The figure shows three views and two pictorial views of one solid part (mm, origin at its lowest corner). Answer the questions. A direction names the side the tool comes from. Coordinates: 2 decimals unless noted, no trailing zeros. Write each loop counter-clockwise with the first axis right and the second up, starting at its lowest first coordinate (ties: lowest second). Pieces come first, ordered by that corner, then holes.
Item 1: A tool of negligible diameter and unlimited length cuts with its end or side. For the marked faces 1 and 2, from which of +Z, -Z, +X, -X, +Y, -Y can it reach the whole face along a straight path? Write none if from no direction.
Item 2: Section C-C (z = 3.5) is taken. Give the vertices of the cut face in (x, y), then the cut area to 3 significant figures.
Item 3: Straight lines are drawn through the part: probe 1 along Y at (x, z) = (3.5, 1.1); probe 2 along X at (y, z) = (12.25, 3) (1 decimal); probe 3 along Z at (x, y) = (3.8, 15.25). For each, find the intervals that lie inside material, in ascending order.
Item 4: Section A-A (y = 9) is taken. Give the vertices of the cut face in (x, z), then the cut area to 3 significant figures.
Item 5: Section D-D (z = 0.4) is taken. Give the vertices of the cut face in (x, y).
Item 6: Section B-B (x = 3) is taken. Give the vertices of the cut face in (y, z).
Item 7: Each of these flat-tipped pins is pushed along its axis until it touches: P1, Ø2.5, axis at x = 3, z = 2.6, coming from the -Y side; P2, Ø1.5, axis at x = 2.5, z = 3, coming from the +Y side. Where does it stop, or does it pass through?
Item 8: Determine the mould class of the marked faces 3, 4 and 5 for opening direction Z: released by +Z, released by -Z, zero draft, split by the parting line, or undercut.
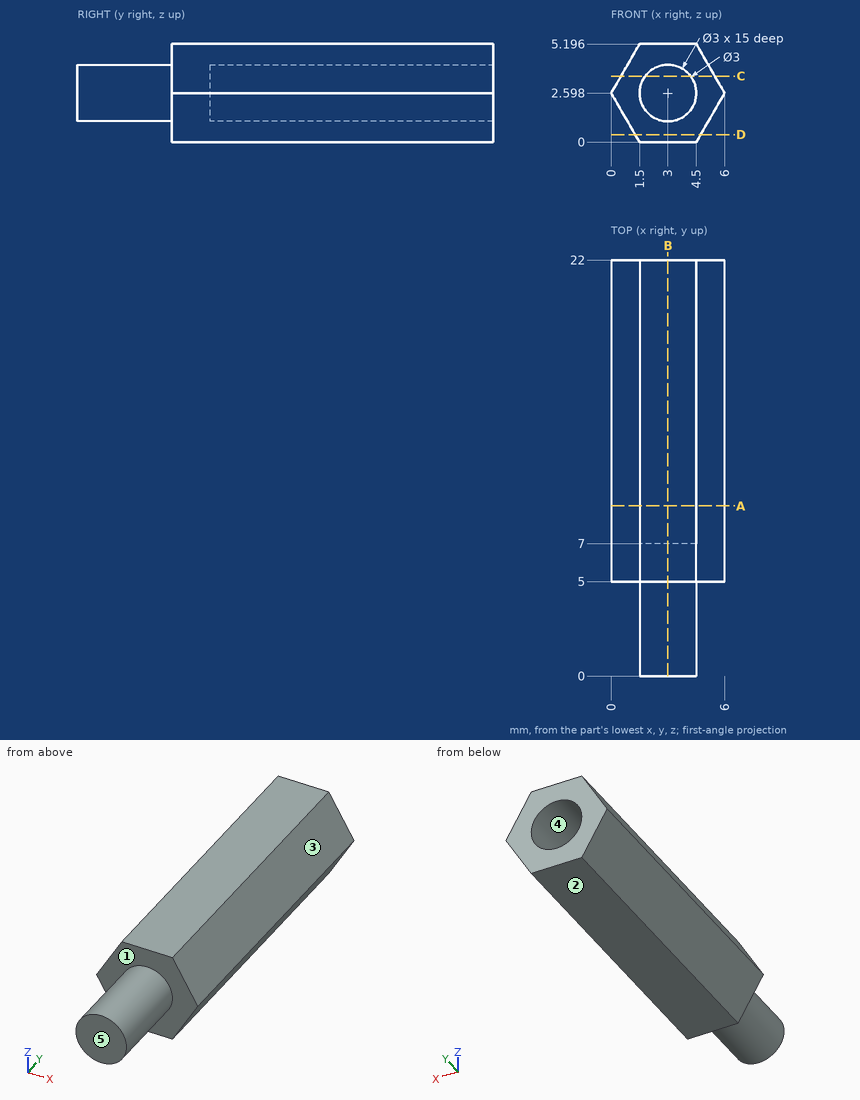
Established:
1. face 1: -Y
1. face 2: -Z, +X, -X, +Y, -Y
2. outline: (0.52, 5) - (1.8, 5) - (1.8, 0) - (4.2, 0) - (4.2, 5) - (5.48, 5) - (5.48, 22) - (4.2, 22) - (4.2, 7) - (1.8, 7) - (1.8, 22) - (0.52, 22) - close
2. area: 60.3 mm2
3. probe 1: y = 5 to 22
3. probe 2: x = 0.2 to 1.6, 4.4 to 5.8
3. probe 3: z = 0 to 1.33, 3.87 to 5.2
4. outline: (0, 2.6) - (1.5, 0) - (4.5, 0) - (6, 2.6) - (4.5, 5.2) - (1.5, 5.2) - close; hole circle Ø3 at (3, 2.6)
4. area: 16.3 mm2
5. outline: (1.27, 5) - (4.73, 5) - (4.73, 22) - (1.27, 22) - close
6. outline: (0, 1.1) - (5, 1.1) - (5, 0) - (22, 0) - (22, 1.1) - (7, 1.1) - (7, 4.1) - (22, 4.1) - (22, 5.2) - (5, 5.2) - (5, 4.1) - (0, 4.1) - close
7. P1: stops at y = 0
7. P2: stops at y = 7
8. face 3: released by +Z
8. face 4: undercut
8. face 5: zero draft
